The listing builds one solid part. Answer for the finished solid, in the listing's coordinates (mm). A direction names the side the tool comes from. Give positions to 0.01 mm unless a question says otherwise; leave off trailing zeros. Order: outer loops, then holes, each group sorted by start corner. A loop starts at its lowest first (then second) coordinate and runs counter-clockwise, first axis right, second up.
```python
from build123d import *

# Parameters (mm, degrees)
SKETCH1_W                                            = 190.5
SKETCH1_H                                            = 152.4
BOSS_EXTRUDE1_DEPTH                                  = 12.7
CBORE_FOR_1_4_BINDING_HEAD_MACHINE_SCREW_D           = 8.3312
CBORE_FOR_1_4_BINDING_HEAD_MACHINE_SCREW_CBORE_D     = 12.7
CBORE_FOR_1_4_BINDING_HEAD_MACHINE_SCREW_CBORE_DEPTH = 8.89
CBORE_FOR_1_4_BINDING_HEAD_MACHINE_S_2_D             = 8.3312
CBORE_FOR_1_4_BINDING_HEAD_MACHINE_S_2_CBORE_D       = 12.7
CBORE_FOR_1_4_BINDING_HEAD_MACHINE_S_2_CBORE_DEPTH   = 8.89
F_3_8_16_TAPPED_HOLE1_D                              = 7.9375
LPATTERN1_COUNT                                      = 2
LPATTERN1_PITCH                                      = 92.075
LPATTERN1_COUNT_DIR2                                 = 2
LPATTERN1_PITCH_DIR2                                 = 66.675


with BuildPart() as part:
    # Sketch1 → Boss-Extrude1 (new body)
    with BuildSketch(Plane(origin=(0, 0, 0), x_dir=(1, 0, 0), z_dir=(0, 1, 0))):
        with Locations((95.25, 76.2)):
            Rectangle(SKETCH1_W, SKETCH1_H)
    extrude(amount=BOSS_EXTRUDE1_DEPTH)

    # CBORE for 1_4 Binding Head Machine Screw (through all)
    with Locations(Plane(origin=(0, 12.7, 0), x_dir=(1, 0, 0), z_dir=(0, 1, 0))):
        with Locations((19.05, 19.05), (57.15, 19.05), (95.25, 19.05), (133.35, 19.05), (19.05, 57.15), (19.05, 95.25), (19.05, 133.35), (57.15, 57.15), (95.25, 57.15), (133.35, 57.15), (57.15, 95.25), (57.15, 133.35)):
            CounterBoreHole(CBORE_FOR_1_4_BINDING_HEAD_MACHINE_SCREW_D / 2, CBORE_FOR_1_4_BINDING_HEAD_MACHINE_SCREW_CBORE_D / 2, CBORE_FOR_1_4_BINDING_HEAD_MACHINE_SCREW_CBORE_DEPTH)

    # CBORE for 1_4 Binding Head Machine S 2 (through all)
    with Locations(Plane(origin=(0, 12.7, 0), x_dir=(1, 0, 0), z_dir=(0, 1, 0))):
        with Locations((171.45, 19.05), (171.45, 57.15)):
            CounterBoreHole(CBORE_FOR_1_4_BINDING_HEAD_MACHINE_S_2_D / 2, CBORE_FOR_1_4_BINDING_HEAD_MACHINE_S_2_CBORE_D / 2, CBORE_FOR_1_4_BINDING_HEAD_MACHINE_S_2_CBORE_DEPTH)

    # 3/8-16 Tapped Hole1 (through all)
    with Locations(Plane(origin=(0, 12.7, 0), x_dir=(1, 0, 0), z_dir=(0, 1, 0))):
        with Locations((17.4625, 41.275)):
            f_3_8_16_tapped_hole1 = Hole(F_3_8_16_TAPPED_HOLE1_D / 2)

    # LPattern1: 3_8-16 Tapped Hole1 2 × 2
    with Locations(*[(i * LPATTERN1_PITCH, 0, -j * LPATTERN1_PITCH_DIR2) for i in range(LPATTERN1_COUNT) for j in range(LPATTERN1_COUNT_DIR2) if (i, j) != (0, 0)]):
        add(f_3_8_16_tapped_hole1, mode=Mode.SUBTRACT)


solid = part.part
```
1) Find section B-B (z = -95.25). Write down the section's boundary in (x, y), then the cut area to 3 significant figures.
Geometry says:
outline: (0, 0) - (14.88, 0) - (14.88, 3.81) - (12.7, 3.81) - (12.7, 12.7) - (0, 12.7) - close; (23.22, 0) - (52.98, 0) - (52.98, 3.81) - (50.8, 3.81) - (50.8, 12.7) - (25.4, 12.7) - (25.4, 3.81) - (23.22, 3.81) - close; (61.32, 0) - (190.5, 0) - (190.5, 12.7) - (63.5, 12.7) - (63.5, 3.81) - (61.32, 3.81) - close
area: 2,130 mm2
2) A tool of negligible diameter and unlimited length cuts with its end or side. For faces 1 (the flat face through (23.2, 3.81, -55.8)), 2 (the cylindrical face through (175.61, 1.88, -19.23)), from which of +Z, -Z, +X, -X, +Y, -Y can it reach the whole face along a straight path? Write none if from no direction.
Geometry says:
face 1: +Y
face 2: +Y, -Y
3) For a pull along X with two mould halves and no side action, classify faces 3 (the flat face through (94, 6, -152.4)), 4 (the cylindrical face through (113.502, 6.261, -108.124)) as +X half, -X half, draft (parallel to the pull), parting line (faces both ways), or undercut.
Geometry says:
face 3: draft
face 4: undercut
4) Find section A-A (x = 133.35). Write down the section's boundary in (y, z), then the cut area to 3 significant figures.
Geometry says:
outline: (0, -152.4) - (12.7, -152.4) - (12.7, -63.5) - (3.81, -63.5) - (3.81, -61.32) - (0, -61.32) - close; (0, -52.98) - (3.81, -52.98) - (3.81, -50.8) - (12.7, -50.8) - (12.7, -25.4) - (3.81, -25.4) - (3.81, -23.22) - (0, -23.22) - close; (0, -14.88) - (3.81, -14.88) - (3.81, -12.7) - (12.7, -12.7) - (12.7, 0) - (0, 0) - close
area: 1,650 mm2
5) Given P1, Ø6.5, axis at x = 19.05, z = -19.05, coming from the -Y side; P2, Ø6.5, axis at x = 17, z = -57, coming from the +Y side, each flat-ended and moving along its own axis, determine where each tip first touches the part or whether it passes through.
Geometry says:
P1: passes through
P2: stops at y = 3.81
6) Straight lines are drawn through the part: probe 1 along X at (y, z) = (6.5, -57.15); probe 2 along X at (y, z) = (2.45, -19.05); probe 3 along Z at (x, y) = (133.35, 2.75). For each, find the intervals that lie inside material, in ascending order.
Geometry says:
probe 1: x = 0 to 12.7, 25.4 to 50.8, 63.5 to 88.9, 101.6 to 127, 139.7 to 165.1, 177.8 to 190.5
probe 2: x = 0 to 14.88, 23.22 to 52.98, 61.32 to 91.08, 99.42 to 129.18, 137.52 to 167.28, 175.62 to 190.5
probe 3: z = -152.4 to -61.32, -52.98 to -23.22, -14.88 to 0
7) Find section C-C (z = -57.15). Count the separate pieces of the cut face and the enclosed holes in it, then the cut area to 3 significant figures.
Geometry says:
separate pieces: 6
enclosed holes: 0
area: 1,700 mm2
